```python
from build123d import *

# Parameters (mm, degrees)
SKETCH_1_R          = 5
EXTRUDE_1_DEPTH     = 46
SKETCH_2_R          = 7
EXTRUDE_2_DEPTH     = 2
CHAMFER_1_SIZE      = 0.5
CUT_EXTRUDE_START   = 2.5
SKETCH_3_R          = 14
SKETCH_3_R_2        = 4
CUT_EXTRUDE_1_DEPTH = 1


with BuildPart() as part:
    # 草图1 → 凸台-拉伸1 (new body)
    with BuildSketch(Plane.XY):
        Circle(SKETCH_1_R)
    extrude(amount=EXTRUDE_1_DEPTH)

    # 草图2 → 凸台-拉伸2 (add)
    with BuildSketch(Plane.XY.offset(46)):
        Circle(SKETCH_2_R)
    extrude(amount=EXTRUDE_2_DEPTH)

    # 倒角1
    chamfer_1_edges = [part.edges().sort_by_distance(p)[0] for p in [
        (-5, 0, 0),
        (-7, 0, 48),
    ]]
    chamfer(chamfer_1_edges, length=CHAMFER_1_SIZE)

    # 草图3 → 切除-拉伸-薄壁1 (cut)
    with BuildSketch(Plane.XY.offset(CUT_EXTRUDE_START)):
        Circle(SKETCH_3_R)
        Circle(SKETCH_3_R_2, mode=Mode.SUBTRACT)
    extrude(amount=CUT_EXTRUDE_1_DEPTH, mode=Mode.SUBTRACT)


solid = part.part
```
Could you check a few things on this model? Use its own coordinates, in mm. A direction names the side the tool comes from. Give positions to 0.01 mm unless a question says otherwise; leave off trailing zeros. Loops run counter-clockwise (first coordinate to the right, second up) from the corner with the lowest first, then second, coordinate; pieces in that order, holes last. Notation, with made-up numbers: (31.25, 47) - (47.25, 47) arc R20 ccw to (47.25, 66) - close; hole circle Ø1 at (32.5, -0.75). An arc over 180 degrees is marked (long way). Answer in a Markdown table with one row per item. Add a question column.
Q1. Which directions (+Z, -Z, +X, -X, +Y, -Y) give clear straight access to the entire face, cutting with the end or side of a thin tool? Please do faces 1 (the face through (0, 0, 48)), 2 (the face through (-2, 5, 46)).
Q2. If we section it at A-A (x = 0): List the corners of the cut face in (y, z) for me.
Q3. We'd pull the mould along Z, two halves only. Please class faces 3 (the face through (6.466, -2.681, 46.74)), 4 (the face through (-0.867, -3.905, 2.993)), 5 (the face through (0, 0, 0)): +Z half, -Z half, draft (parallel to the pull), parting line (faces both ways), or undercut.
Q4. If we section it at C-C (z = 7.5): List the corners of the cut face in (x, y) for me.
Q5. Please list where these lines run through material, in increasing order: L1, parallel to Z at x = 1.5, y = -4; L2, parallel to Z at x = -4.5, y = 2.75; L3, parallel to X at y = 0.25, z = 7.5. Write a range as from..to.
Q6. For pin 1 (3 mm diameter, centred on x = -1.5, y = 0, fed in from -Z); pin 2 (1 mm diameter, centred on x = 0, z = 24, fed in from +Y); pin 3 (6 mm diameter, centred on y = -1.5, z = 16.5, fed in from -X); pin 4 (3 mm diameter, centred on x = 3.5, z = 34, fed in from +Y), each with a flat end and sliding along its axis, tell me the tip position at first contact or that it passes through.
The answers:
| question | item | result |
|---|---|---|
| 1 | face 1 | +Z, +X, -X, +Y, -Y |
| 1 | face 2 | -Z |
| 2 | outline | (-7, 46) - (-5, 46) - (-5, 3.5) - (-4, 3.5) - (-4, 2.5) - (-5, 2.5) - (-5, 0.5) - (-4.5, 0) - (4.5, 0) - (5, 0.5) - (5, 2.5) - (4, 2.5) - (4, 3.5) - (5, 3.5) - (5, 46) - (7, 46) - (7, 47.5) - (6.5, 48) - (-6.5, 48) - (-7, 47.5) - close |
| 3 | face 3 | draft |
| 3 | face 4 | undercut |
| 3 | face 5 | -Z half |
| 4 | outline | circle Ø10 at (0, 0) |
| 5 | L1 | z = 0..2.5, 3.5..48 |
| 5 | L2 | z = 46..48 |
| 5 | L3 | x = -4.99..4.99 |
| 6 | pin 1 | stops at z = 0 |
| 6 | pin 2 | stops at y = 5 |
| 6 | pin 3 | stops at x = -5 |
| 6 | pin 4 | stops at y = 4.58 |
